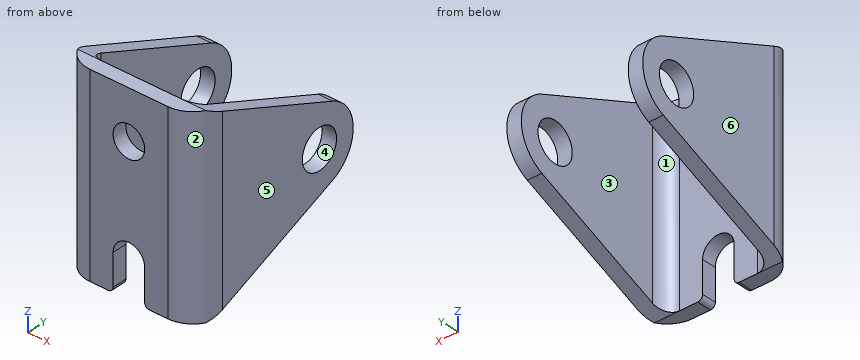
from build123d import *

# Parameters (mm, degrees)
SKETCH1_R           = 3.25
BOSS_EXTRUDE1_DEPTH = 3
SKETCH2_R           = 4.05
BOSS_EXTRUDE2_DEPTH = 3
FILLET1_R           = 6
FILLET2_R           = 3


with BuildPart() as part:
    # Sketch1 → Boss-Extrude1 (new body)
    with BuildSketch(Plane(origin=(0, 0, 0), x_dir=(1, 0, 0), z_dir=(0, 1, 0))):
        with BuildLine():
            Line((-11, -19.75), (11, -19.75))
            Line((11, -19.75), (11, 19.75))
            Line((11, 19.75), (4.25, 19.75))
            ThreePointArc((4.25, 19.75), (3.542893219, 19.457106781), (3.25, 18.75))
            Line((3.25, 18.75), (3.25, 12.25))
            ThreePointArc((3.25, 12.25), (0, 9), (-3.25, 12.25))
            Line((-3.25, 12.25), (-3.25, 18.75))
            ThreePointArc((-3.25, 18.75), (-3.542893219, 19.457106781), (-4.25, 19.75))
            Line((-4.25, 19.75), (-11, 19.75))
            Line((-11, 19.75), (-11, -19.75))
        make_face()
        with Locations(Location((0, -9.75, 0), (0, 0, 270))):
            Circle(SKETCH1_R, mode=Mode.SUBTRACT)
    extrude(amount=BOSS_EXTRUDE1_DEPTH)

    # Sketch2 → Boss-Extrude2 (add)
    with BuildSketch(Plane(origin=(11, 0, 0), x_dir=(0, 0, -1), z_dir=(1, 0, 0))):
        with BuildLine():
            Line((-19.75, 3), (-7.361967169, 32.130725061))
            ThreePointArc((-7.361967169, 32.130725061), (0, 37), (7.361967169, 32.130725061))
            Line((7.361967169, 32.130725061), (19.75, 3))
            Line((19.75, 3), (19.75, 0))
            Line((19.75, 0), (-19.75, 0))
            Line((-19.75, 0), (-19.75, 3))
        make_face()
        with Locations((0, 29)):
            Circle(SKETCH2_R, mode=Mode.SUBTRACT)
    boss_extrude2 = extrude(amount=BOSS_EXTRUDE2_DEPTH)

    # Mirror1: Boss-Extrude2 across plane
    add(boss_extrude2.mirror(Plane(origin=(0, 0, 0), x_dir=(0, 0, 1), z_dir=(1, 0, 0))))

    # Fillet1
    fillet1_edges = [part.edges().sort_by_distance(p)[0] for p in [
        (-14, 0, 0),
        (14, 0, 0),
    ]]
    fillet(fillet1_edges, radius=FILLET1_R)

    # Fillet2
    fillet2_edges = [part.edges().sort_by_distance(p)[0] for p in [
        (-11, 3, 0),
        (11, 3, 0),
    ]]
    fillet(fillet2_edges, radius=FILLET2_R)


solid = part.part
The model under review builds one solid part; all positions refer to its coordinate system, in mm. Face numbers are marked on the shaded views. A direction names the side the tool comes from. Coordinates: 2 decimals unless noted, no trailing zeros. Write each loop counter-clockwise with the first axis right and the second up, starting at its lowest first coordinate (ties: lowest second). Pieces come first, ordered by that corner, then holes. Notation, with made-up numbers: (5.25, 14.25) - (42.25, 14.25) arc R31 cw to (42.25, 47.25) - close; hole circle Ø7 at (89, 7.25). An arc over 180 degrees is marked (long way). Answer as CSV lines item,"result".
(1) We need section A-A (z = 0). Give the boundary of the cut face in (x, y), plus the area to 3 significant figures.
Data:
outline,"(-14, 6) arc R6 ccw to (-8, 0) - (8, 0) arc R6 ccw to (14, 6) - (14, 24.95) - (11, 24.95) - (11, 6) arc R3 cw to (8, 3) - (-8, 3) arc R3 cw to (-11, 6) - (-11, 24.95) - (-14, 24.95) - close; (-14, 33.05) - (-11, 33.05) - (-11, 37) - (-14, 37) - close; (11, 33.05) - (14, 33.05) - (14, 37) - (11, 37) - close"
area,"228 mm2"
(2) Tool access review of the marked faces 1 and 2: name each direction out of +Z, -Z, +X, -X, +Y, -Y from which nothing blocks a thin tool from reaching the whole face with its end or side.
Data:
face 1,"+Z, -Z, +Y"
face 2,"+Z, -Z, +X, -Y"
(3) We need section B-B (y = 3.5). Give the boundary of the cut face in (x, z), plus the area to 3 significant figures.
Data:
outline,"(-13.45, -19.54) - (-9.66, -19.54) - (-9.66, 19.54) - (-13.45, 19.54) - close; (9.66, -19.54) - (13.45, -19.54) - (13.45, 19.54) - (9.66, 19.54) - close"
area,"297 mm2"
(4) We need section D-D (z = 9.75). Give the boundary of the cut face in (x, y), plus the area to 3 significant figures.
Data:
outline,"(-14, 6) arc R6 ccw to (-8, 0) - (-3.25, 0) - (-3.25, 3) - (-8, 3) arc R3 cw to (-11, 6) - (-11, 26.52) - (-14, 26.52) - close; (3.25, 0) - (8, 0) arc R6 ccw to (14, 6) - (14, 26.52) - (11, 26.52) - (11, 6) arc R3 cw to (8, 3) - (3.25, 3) - close"
area,"194 mm2"
(5) Mouldability with a two-part tool opening along X and no side actions: class the marked faces 3, 4, 5 and 6 as pulls with the +X half, pulls with the -X half, needs draft (parallel to the pull), parting line crosses it, or undercut.
Data:
face 3,"undercut"
face 4,"needs draft"
face 5,"pulls with the +X half"
face 6,"pulls with the -X half"
(6) We need section C-C (x = 0). Give the boundary of the cut face in (y, z).
Data:
outline,"(0, -9) - (3, -9) - (3, 6.5) - (0, 6.5) - close; (0, 13) - (3, 13) - (3, 19.75) - (0, 19.75) - close"
(7) For line 1 along X through (y, z) = (12, -13); line 2 along X through (y, z) = (1.8, 9.75); line 3 along Y through (x, z) = (-5.75, 15), list the stretches that pass through material, from the lowest coordinate up. Write a range as [from, to].
Data:
line 1,"x = [-14, -11], [11, 14]"
line 2,"x = [-12.28, -3.25], [3.25, 12.28]"
line 3,"y = [0, 3]"
(8) Clearance check with flat-ended pins moving along their axes: pin 1 Ø3 at (x, z) = (2.5, -2) entering from +Y; pin 2 Ø0.9 at (y, z) = (1.5, -15) entering from +X; pin 3 Ø13 at (x, z) = (3.5, 7.5) entering from +Y. State where each tip first meets the part, or that it passes through.
Data:
pin 1,"stops at y = 3"
pin 2,"stops at x = 12.43"
pin 3,"stops at y = 3.76"
